from build123d import *

# Parameters (mm, degrees)
EXTRUDE_1_DEPTH     = 5
SKETCH_2_R          = 25.5
SKETCH_2_R_2        = 17
CUT_EXTRUDE_1_DEPTH = 3.2
CUT_EXTRUDE_2_DEPTH = 18.2
FILLET_1_R          = 2
SKETCH_4_W          = 1.7
SKETCH_4_H          = 1.7
CUT_EXTRUDE_3_DEPTH = 71
SKETCH_5_R          = 1.65
CUT_EXTRUDE_4_DEPTH = 3
SKETCH_6_W          = 10
SKETCH_6_H          = 7.8
CUT_EXTRUDE_5_DEPTH = 9.4


with BuildPart() as part:
    # Эскиз1 → Бобышка-Вытянуть1 (new body)
    with BuildSketch(Plane(origin=(0, 0, 0), x_dir=(1, 0, 0), z_dir=(0, 1, 0))):
        with BuildLine():
            Line((-52.404740413, 37.47648532), (56.595259587, 37.47648532))
            ThreePointArc((56.595259587, 37.47648532), (58.716579931, 36.597805664), (59.595259587, 34.47648532))
            Line((59.595259587, 34.47648532), (59.595259587, -14.52351468))
            ThreePointArc((59.595259587, -14.52351468), (58.716579931, -16.644835023), (56.595259587, -17.52351468))
            Line((56.595259587, -17.52351468), (-52.404740413, -17.52351468))
            ThreePointArc((-52.404740413, -17.52351468), (-54.526060756, -16.644835023), (-55.404740413, -14.52351468))
            Line((-55.404740413, -14.52351468), (-55.404740413, 34.47648532))
            ThreePointArc((-55.404740413, 34.47648532), (-54.526060756, 36.597805664), (-52.404740413, 37.47648532))
        make_face()
    extrude(amount=EXTRUDE_1_DEPTH)

    # Эскиз2 → Вырез-Вытянуть1 (cut)
    with BuildSketch(Plane(origin=(0, 5, 0), x_dir=(1, 0, 0), z_dir=(0, 1, 0))):
        with Locations(Location((2.095259587, 9.97648532, 0), (0, 0, 270))):
            Circle(SKETCH_2_R)
        with Locations(Location((2.095259587, 9.97648532, 0), (0, 0, 270))):
            Circle(SKETCH_2_R_2, mode=Mode.SUBTRACT)
    extrude(amount=-CUT_EXTRUDE_1_DEPTH, mode=Mode.SUBTRACT)

    # Эскиз3 → Вырез-Вытянуть2 (cut)
    with BuildSketch(Plane(origin=(0, 5, 0), x_dir=(1, 0, 0), z_dir=(0, 1, 0))):
        with BuildLine():
            Line((-45.404740413, 32.47648532), (-44.404740413, 32.47648532))
            ThreePointArc((-44.404740413, 32.47648532), (-42.99052685, 31.890698883), (-42.404740413, 30.47648532))
            Line((-42.404740413, 30.47648532), (-42.404740413, -10.52351468))
            ThreePointArc((-42.404740413, -10.52351468), (-42.99052685, -11.937728242), (-44.404740413, -12.52351468))
            Line((-44.404740413, -12.52351468), (-45.404740413, -12.52351468))
            ThreePointArc((-45.404740413, -12.52351468), (-46.818953975, -11.937728242), (-47.404740413, -10.52351468))
            Line((-47.404740413, -10.52351468), (-47.404740413, 30.47648532))
            ThreePointArc((-47.404740413, 30.47648532), (-46.818953975, 31.890698883), (-45.404740413, 32.47648532))
        make_face()
        with BuildLine():
            Line((-37.404740413, 32.47648532), (-36.404740413, 32.47648532))
            ThreePointArc((-36.404740413, 32.47648532), (-34.99052685, 31.890698883), (-34.404740413, 30.47648532))
            Line((-34.404740413, 30.47648532), (-34.404740413, -10.52351468))
            ThreePointArc((-34.404740413, -10.52351468), (-34.99052685, -11.937728242), (-36.404740413, -12.52351468))
            Line((-36.404740413, -12.52351468), (-37.404740413, -12.52351468))
            ThreePointArc((-37.404740413, -12.52351468), (-38.818953975, -11.937728242), (-39.404740413, -10.52351468))
            Line((-39.404740413, -10.52351468), (-39.404740413, 30.47648532))
            ThreePointArc((-39.404740413, 30.47648532), (-38.818953975, 31.890698883), (-37.404740413, 32.47648532))
        make_face()
        with BuildLine():
            Line((-29.404740413, 32.47648532), (-28.404740413, 32.47648532))
            ThreePointArc((-28.404740413, 32.47648532), (-26.99052685, 31.890698883), (-26.404740413, 30.47648532))
            Line((-26.404740413, 30.47648532), (-26.404740413, -10.52351468))
            ThreePointArc((-26.404740413, -10.52351468), (-26.99052685, -11.937728242), (-28.404740413, -12.52351468))
            Line((-28.404740413, -12.52351468), (-29.404740413, -12.52351468))
            ThreePointArc((-29.404740413, -12.52351468), (-30.818953975, -11.937728242), (-31.404740413, -10.52351468))
            Line((-31.404740413, -10.52351468), (-31.404740413, 30.47648532))
            ThreePointArc((-31.404740413, 30.47648532), (-30.818953975, 31.890698883), (-29.404740413, 32.47648532))
        make_face()
        with BuildLine():
            Line((49.595259587, 32.47648532), (48.595259587, 32.47648532))
            ThreePointArc((48.595259587, 32.47648532), (47.181046025, 31.890698883), (46.595259587, 30.47648532))
            Line((46.595259587, 30.47648532), (46.595259587, -10.52351468))
            ThreePointArc((46.595259587, -10.52351468), (47.181046025, -11.937728242), (48.595259587, -12.52351468))
            Line((48.595259587, -12.52351468), (49.595259587, -12.52351468))
            ThreePointArc((49.595259587, -12.52351468), (51.00947315, -11.937728242), (51.595259587, -10.52351468))
            Line((51.595259587, -10.52351468), (51.595259587, 30.47648532))
            ThreePointArc((51.595259587, 30.47648532), (51.00947315, 31.890698883), (49.595259587, 32.47648532))
        make_face()
        with BuildLine():
            Line((41.595259587, 32.47648532), (40.595259587, 32.47648532))
            ThreePointArc((40.595259587, 32.47648532), (39.181046025, 31.890698883), (38.595259587, 30.47648532))
            Line((38.595259587, 30.47648532), (38.595259587, -10.52351468))
            ThreePointArc((38.595259587, -10.52351468), (39.181046025, -11.937728242), (40.595259587, -12.52351468))
            Line((40.595259587, -12.52351468), (41.595259587, -12.52351468))
            ThreePointArc((41.595259587, -12.52351468), (43.00947315, -11.937728242), (43.595259587, -10.52351468))
            Line((43.595259587, -10.52351468), (43.595259587, 30.47648532))
            ThreePointArc((43.595259587, 30.47648532), (43.00947315, 31.890698883), (41.595259587, 32.47648532))
        make_face()
        with BuildLine():
            Line((33.595259587, 32.47648532), (32.595259587, 32.47648532))
            ThreePointArc((32.595259587, 32.47648532), (31.181046025, 31.890698883), (30.595259587, 30.47648532))
            Line((30.595259587, 30.47648532), (30.595259587, -10.52351468))
            ThreePointArc((30.595259587, -10.52351468), (31.181046025, -11.937728242), (32.595259587, -12.52351468))
            Line((32.595259587, -12.52351468), (33.595259587, -12.52351468))
            ThreePointArc((33.595259587, -12.52351468), (35.00947315, -11.937728242), (35.595259587, -10.52351468))
            Line((35.595259587, -10.52351468), (35.595259587, 30.47648532))
            ThreePointArc((35.595259587, 30.47648532), (35.00947315, 31.890698883), (33.595259587, 32.47648532))
        make_face()
    extrude(amount=-CUT_EXTRUDE_2_DEPTH, mode=Mode.SUBTRACT)

    # Скругление1
    fillet_1_edges = [part.edges().sort_by_distance(p)[0] for p in [
        (58.716579931, 5, 16.644835023),
        (59.595259587, 5, -9.97648532),
        (58.716579931, 5, -36.597805664),
        (2.095259587, 5, -37.47648532),
        (-54.526060756, 5, -36.597805664),
        (-55.404740413, 5, -9.97648532),
        (-54.526060756, 5, 16.644835023),
        (2.095259587, 5, 17.52351468),
    ]]
    fillet(fillet_1_edges, radius=FILLET_1_R - 0.0001)  # a hair under: the kernel refuses the full size

    # Эскиз4 → Вырез-Вытянуть3 (cut)
    with BuildSketch(Plane.XZ):
        with Locations((-51.554740413, 13.67351468)):
            Rectangle(SKETCH_4_W, SKETCH_4_H)
        with Locations((-51.554740413, -33.62648532)):
            Rectangle(SKETCH_4_W, SKETCH_4_H)
        with Locations((55.745259587, -33.62648532)):
            Rectangle(SKETCH_4_W, SKETCH_4_H)
        with Locations((55.745259587, 13.67351468)):
            Rectangle(SKETCH_4_W, SKETCH_4_H)
    extrude(amount=-CUT_EXTRUDE_3_DEPTH, mode=Mode.SUBTRACT)

    # Эскиз5 → Вырез-Вытянуть4 (cut)
    with BuildSketch(Plane(origin=(0, 5, 0), x_dir=(1, 0, 0), z_dir=(0, 1, 0))):
        with Locations(Location((-51.554740413, 33.62648532, 0), (0, 0, 270))):
            Circle(SKETCH_5_R)
        with Locations(Location((-51.554740413, -13.67351468, 0), (0, 0, 270))):
            Circle(SKETCH_5_R)
        with Locations(Location((55.745259587, 33.62648532, 0), (0, 0, 270))):
            Circle(SKETCH_5_R)
        with Locations(Location((55.745259587, -13.67351468, 0), (0, 0, 270))):
            Circle(SKETCH_5_R)
    extrude(amount=-CUT_EXTRUDE_4_DEPTH, mode=Mode.SUBTRACT)

    # Эскиз6 → Вырез-Вытянуть5 (cut)
    with BuildSketch(Plane(origin=(0, 1.8, 0), x_dir=(1, 0, 0), z_dir=(0, 1, 0))):
        with Locations((2.095259587, 31.57648532)):
            Rectangle(SKETCH_6_W, SKETCH_6_H)
    extrude(amount=-CUT_EXTRUDE_5_DEPTH, mode=Mode.SUBTRACT)


solid = part.part
Design review of the part built by this model. Coordinates are the model's own, in mm. A direction names the side the tool comes from. Round coordinates to 2 decimals unless told otherwise and drop trailing zeros. Loops run counter-clockwise (first coordinate to the right, second up) from the corner with the lowest first, then second, coordinate; pieces in that order, holes last. Notation, with made-up numbers: (34, -8.75) - (75, -8.75) arc R18 cw to (75, -3.75) - close; hole circle Ø11 at (2.5, 71). An arc over 180 degrees is marked (long way). One line per question, with ' | ' between items.
1. We need section C-C, the plane x = 14.5. State the section outline as (y, z) points.
Results are:
outline: (0, -37.48) - (3, -37.48) arc R2 ccw to (5, -35.48) - (5, -32.26) - (1.8, -32.26) - (1.8, -21.6) - (5, -21.6) - (5, 1.65) - (1.8, 1.65) - (1.8, 12.3) - (5, 12.3) - (5, 15.52) arc R2 ccw to (3, 17.52) - (0, 17.52) - close
2. For faces 4 (the face through (-52.187, 3.521, -32.102)), 5 (the face through (3, 1, 17.524)), 6 (the face through (-30.83, 2.54, -31.88)), list the 3-axis set-ups (+Z, -Z, +X, -X, +Y, -Y) from which the entire face can be reached by the end or side of a thin tool; tool diameter is ignored.
Results are:
face 4: +Y | face 5: +Z, +X, -X, +Y, -Y | face 6: +Y, -Y
3. For L1, parallel to Z at x = -45.5, y = 2.4; L2, parallel to Z at x = 8.5, y = 2.65; L3, parallel to Z at x = 3.5, y = 2, list the stretches that pass through material, from the lowest coordinate up. Write a range as [from, to].
Results are:
L1: z = [-37.48, -32.47], [12.52, 17.52] | L2: z = [-37.48, -34.66], [-25.72, 5.77], [14.71, 17.52] | L3: z = [-37.48, -35.44], [-26.92, 6.97], [15.48, 17.52]
4. Draft analysis for pull direction X (two halves, no side actions). For faces 1 (the face through (58.994, 4.43, -9.633)), 2 (the face through (2, 5, -10)), 3 (the face through (43.595, 3, -10)), state which applies: released by +X, released by -X, zero draft, split by the parting line, or undercut.
Results are:
face 1: released by +X | face 2: zero draft | face 3: undercut
5. Clearance check with flat-ended pins moving along their axes: P1, Ø1.5, axis at x = 31.5, y = 4.5, coming from the -Z side; P2, Ø1.5, axis at x = -15, y = 4.5, coming from the +Z side. State where each tip first meets the part, or that it passes through.
Results are:
P1: stops at z = -37.33 | P2: stops at z = 17.38
6. We need section A-A, the plane z = 9. State how many separate pieces and enclosed holes the cut face has, and give its area (3 significant figures).
Results are:
separate pieces: 7 | enclosed holes: 0 | area: 314 mm²
